from build123d import *


with BuildPart() as part:
    # Skizze1 → Basis-Rotation (revolve)
    with BuildSketch(Plane.XY, mode=Mode.PRIVATE) as basis_rotation_sk:
        with BuildLine():
            Line((-6, -11), (-7, -11))
            Line((-7, -11), (-7, -1))
            ThreePointArc((-7, -1), (-7.292893219, -0.292893219), (-8, 0))
            Line((-8, 0), (-10, 0))
            Line((-10, 0), (-10, 1))
            Line((-10, 1), (-8, 1))
            ThreePointArc((-8, 1), (-6.585786438, 0.414213562), (-6, -1))
            Line((-6, -1), (-6, -11))
        make_face()
    revolve(basis_rotation_sk.sketch.rotate(Axis((0, 7.790971461, 0), (0, -1, 0)), 270), axis=Axis((0, 7.790971461, 0), (0, -1, 0)))


solid = part.part
Could you check a few things on this model? Use its own coordinates, in mm. A direction names the side the tool comes from. Coordinates: 2 decimals unless noted, no trailing zeros. Write each loop counter-clockwise with the first axis right and the second up, starting at its lowest first coordinate (ties: lowest second). Pieces come first, ordered by that corner, then holes. Notation, with made-up numbers: (55, 87.5) - (99, 87.5) arc R36 ccw to (99, 124.5) - close; hole circle Ø2 at (69.25, 64.25). An arc over 180 degrees is marked (long way). Write item = value, one per line.
1) Suppose I cut it at C-C on y = -4.25. Please give me the cut outline in (x, z).
Result set:
outline = circle Ø14 at (0, 0); hole circle Ø12 at (0, 0)
2) We'd pull the mould along Z, two halves only. Please class faces 1 (the cylindrical face through (-1.802, -6.07, 5.723)), 2 (the flat face through (-2, -11, -6)), 3 (the cylindrical face through (9.76, 0.51, -2.17)): +Z half, -Z half, draft (parallel to the pull), parting line (faces both ways), or undercut.
Result set:
face_1 = undercut
face_2 = draft
face_3 = parting line
3) Please list where these lines run through material, in increasing order: line 1 (X direction, y = -2.75, z = 0); line 2 (Z direction, x = -0.25, y = -5.5); line 3 (Y direction, x = -8.5, z = -3.5). Write a range as [from, to].
Result set:
line_1 = [-7, -6], [6, 7]
line_2 = [-7, -5.99], [5.99, 7]
line_3 = [0, 1]
4) Suppose I cut it at D-D on z = 8.25. Please give me the cut outline in (x, y), plus the area to 3 significant figures.
Result set:
outline = (-5.65, 0) - (5.65, 0) - (5.65, 1) - (-5.65, 1) - close
area = 11.3 mm2
5) Suppose I cut it at B-B on z = 0. Please give me the cut outline in (x, y).
Result set:
outline = (-10, 0) - (-8, 0) arc R1 cw to (-7, -1) - (-7, -11) - (-6, -11) - (-6, -1) arc R2 ccw to (-8, 1) - (-10, 1) - close; (6, -11) - (7, -11) - (7, -1) arc R1 cw to (8, 0) - (10, 0) - (10, 1) - (8, 1) arc R2 ccw to (6, -1) - close
6) Suppose I cut it at A-A on x = 0. Please give me the cut outline in (y, z).
Result set:
outline = (-11, -7) - (-1, -7) arc R1 cw to (0, -8) - (0, -10) - (1, -10) - (1, -8) arc R2 ccw to (-1, -6) - (-11, -6) - close; (-11, 6) - (-1, 6) arc R2 ccw to (1, 8) - (1, 10) - (0, 10) - (0, 8) arc R1 cw to (-1, 7) - (-11, 7) - close
7) For faces 4 (the cylindrical face through (6.834, -5.93, -1.517)), 5 (the flat face through (-8.2, 1, 0)), which set-ups out of +Z, -Z, +X, -X, +Y, -Y let a thin tool reach every point of the face, with its end or its side?
Result set:
face_4 = -Y
face_5 = +Z, -Z, +X, -X, +Y
8) Will these pins go through, and if not, where does the flat tip stop? pin 1 Ø1 at (x, z) = (1.5, -4.5) entering from -Y; pin 2 Ø1.5 at (y, z) = (-0.5, 4) entering from -X; pin 3 Ø1 at (y, z) = (-8.5, 3.5) entering from -X.
Result set:
pin_1 = through
pin_2 = -9.39
pin_3 = -6.32
